Part print with two shaded views. Sizes in mm from the minimum x, y, z corner. A direction names the side the tool comes from. Round coordinates to 2 decimals unless told otherwise and drop trailing zeros. Loops run counter-clockwise (first coordinate to the right, second up) from the corner with the lowest first, then second, coordinate; pieces in that order, holes last. Notation, with made-up numbers: (5.5, 62) - (12.5, 62) arc R29 cw to (12.5, 97) - close; hole circle Ø11 at (-31, 37). An arc over 180 degrees is marked (long way). Write each question's results on one line, items separated by ' | '. Start each with the question number.
(1) Cut at C-C, the plane x = 12.5. List the corners of the cut face in (y, z).
(2) Cut at B-B, the plane z = 5.25. List the corners of the cut face in (x, y), then the cut area to 3 significant figures.
(3) Flat gauge pin, fed straight in: P1, Ø2, axis at x = 9, y = 5.5, coming from the -Z side. Where does the tip first touch, or does it go through?
(4) Tool access for the marked faces 1, 2 and 3: list every direction of +Z, -Z, +X, -X, +Y, -Y with a clear straight run to the whole face (end or side of a thin tool).
(5) Drill centre lines: L1, parallel to Y at x = 14.5, z = 3.5 (1 decimal); L2, parallel to Y at x = 4.5, z = 1.25 (1 decimal); L3, parallel to Z at x = 7, y = 6.25 (1 decimal). Where is each one in solid material? Low to high.
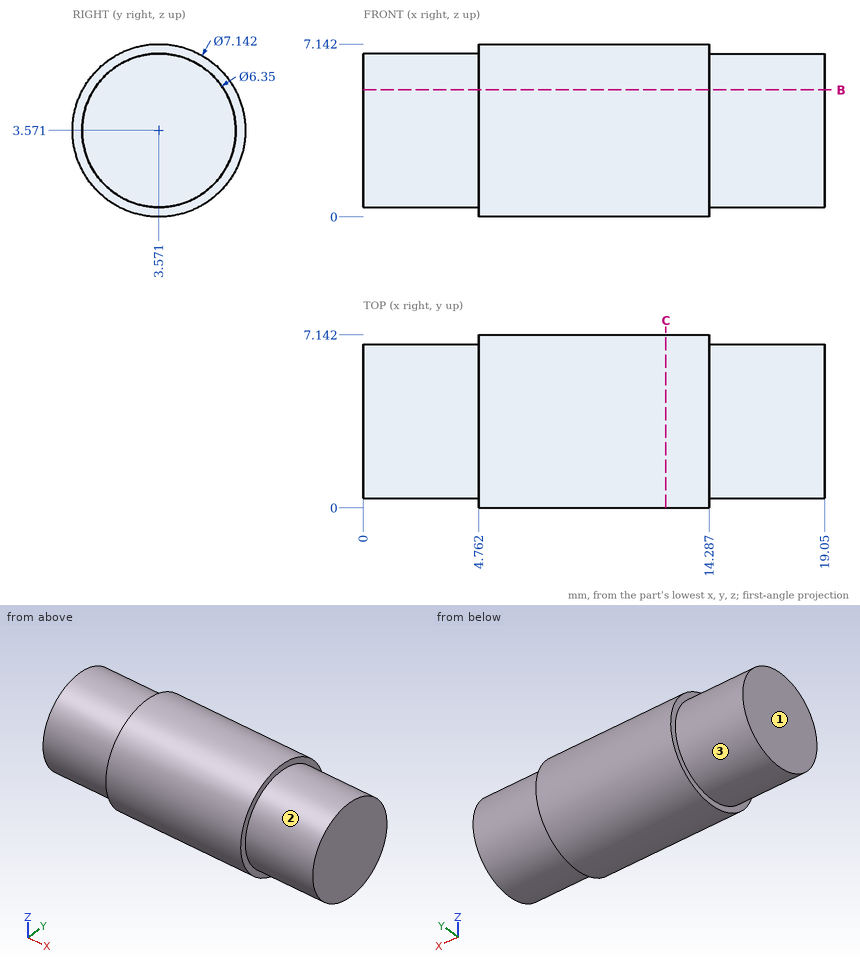
A:
1) outline: circle Ø7.14 at (3.57, 3.57)
2) outline: (0, 0.88) - (4.76, 0.88) - (4.76, 0.42) - (14.29, 0.42) - (14.29, 0.88) - (19.05, 0.88) - (19.05, 6.27) - (14.29, 6.27) - (14.29, 6.72) - (4.76, 6.72) - (4.76, 6.27) - (0, 6.27) - close | area: 111 mm2
3) P1: z = 0.12
4) face 1: +Z, -Z, -X, +Y, -Y | face 2: +X | face 3: -X
5) L1: 0.4 to 6.7 | L2: 1.4 to 5.7 | L3: 1.2 to 5.9
